Check sheet for the modelled part. Datum: model origin and axes. Units: mm. Face numbers are marked on the shaded views. A direction names the side the tool comes from. Coordinates: 2 decimals unless noted, no trailing zeros. Loops run counter-clockwise (first coordinate to the right, second up) from the corner with the lowest first, then second, coordinate; pieces in that order, holes last. Notation, with made-up numbers: (-21.5, -26.75) - (18.5, -26.75) arc R26 cw to (18.5, -2.75) - close; hole circle Ø4 at (78.5, -36.5). An arc over 180 degrees is marked (long way). Use a Markdown table: item, result. Add a question column.
1) Sectioned sample at C-C, the plane y = 41.5. Enter the section's corners in (x, z) (3 decimals), then the cut area to 3 significant figures.
2) Sectioned sample at D-D, the plane z = 34. Enter the section's corners in (x, y) (3 decimals), then the cut area to 3 significant figures.
3) Thickness scan on line 1 (Y direction, x = 21.5, z = 5); line 2 (Z direction, x = 13.75, y = 14) (3 decimals); line 3 (X direction, y = 38.5, z = 10) (3 decimals). Record the ranges inside material, lowest first.
4) Go/stop test with flat-tipped pins: P1, Ø5, axis at y = 5, z = 23.5, coming from the -X side; P2, Ø12, axis at y = 36, z = 15, coming from the +X side (3 decimals); P3, Ø12.5, axis at x = 15.5, y = 23, coming from the +Z side; P4, Ø1.6, axis at y = -2, z = 38, coming from the +X side (3 decimals). Record where each tip stops, or that it passes through.
5) Sectioned sample at B-B, the plane z = 51. Enter the section's corners in (x, y) (3 decimals), then the cut area to 3 significant figures.
6) Tool access check on the marked faces 1 and 2. Record the directions out of +Z, -Z, +X, -X, +Y, -Y that give a thin tool (end or side, any length) a straight path to the whole face; none if there is none.
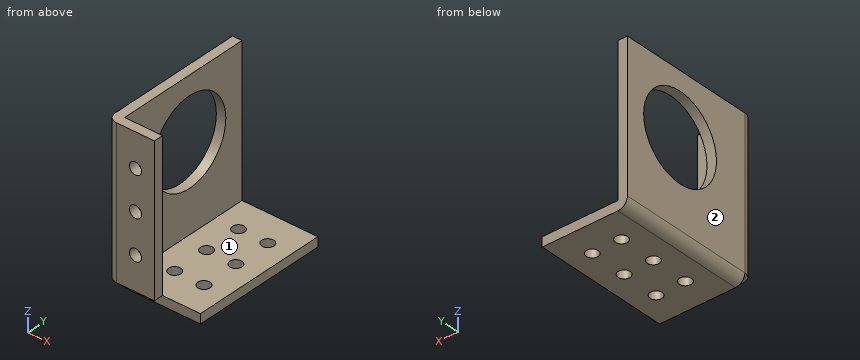
Autodesk Inventor part; units mm, degrees
ref_plane "YZ Plane" through (0, 0, 0) normal (1, 0, 0) x (0, 1, 0)
ref_plane "XZ Plane" through (0, 0, 0) normal (0, 1, 0) x (-1, 0, 0)
ref_plane "XY Plane" through (0, 0, 0) normal (0, 0, 1) x (1, 0, 0)
sketch "Sketch1" plane through (0, 0, 0) normal (1, 0, 0) x (0, 1, 0)
  line L0 (0, 0) -> (46.0357, 0)
  line L1 (46.0357, 0) -> (46.0357, -49.1998)
  line L2 (46.0357, -49.1998) -> (0, -49.1998)
  line L3 (0, -49.1998) -> (0, 0)
  circle A0 centre (25.4109, -28.575) radius 14.2748
  point P0 (39.6857, -28.575)
  point P1 (25.4109, -42.8498)
  dimension "d0" = 25.4109
  dimension "d1" = 28.5496
  dimension "d2" = 6.35
  dimension "d3" = 6.35
  dimension "d4" = 28.575
extrude "Extrusion1" add sketch "Sketch1" along normal blind 3.175
sketch "Sketch2" plane through (0, 0, -49.1998) normal (0, -1, 0) x (1, 0, 0)
  line L0 (3.175, 49.1998) -> (3.175, 0)
  line L1 (3.175, 49.1998) -> (15.875, 49.1998)
  line L2 (15.875, 49.1998) -> (15.875, 0)
  line L3 (15.875, 0) -> (3.175, 0)
  line L4 (3.175, 0) -> (3.175, 49.1998)
  point P0 (0, 49.1998)
  dimension "d7" = 12.7
extrude "Extrusion2" add sketch "Sketch2" along normal blind 3.175
sketch "Sketch3" plane through (0, 0, 0) normal (0, 0, 1) x (1, 0, 0)
  line L0 (3.175, 0) -> (3.175, 46.0357)
  line L1 (3.175, 0) -> (28.575, 0)
  line L2 (28.575, 0) -> (28.575, 49.2107)
  line L3 (28.575, 49.2107) -> (3.175, 49.2107)
  line L4 (3.175, 49.2107) -> (3.175, 0)
  point P0 (0, 0)
  dimension "d10" = 25.4
extrude "Extrusion3" add sketch "Sketch3" along normal blind 3.175
sketch "Sketch4" plane through (3.175, -3.175, 0) normal (0, 0, 1) x (1, 0, 0)
  line L0 (-3.175, 3.175) -> (0, 3.175)
  line L1 (0, 3.175) -> (0, 0)
  arc A0 (-3.175, 3.175) -> (0, 0) centre (0, 3.175) ccw
extrude "Extrusion4" add sketch "Sketch4" against normal up to surface (49.1998 mm away)
sketch "Sketch6" plane through (0, 0, 3.175) normal (0, 0, 1) x (1, 0, 0)
  line L0 (3.175, 0) -> (28.575, 0)
  line L1 (28.575, 0) -> (28.575, 49.2107)
  line L2 (28.575, 49.2107) -> (3.175, 49.2107)
  circle A0 centre (10.9643, 35.5428) radius 2.032
  circle A1 centre (20.7857, 35.5428) radius 2.032
  line L3 (12.9963, 35.5428) -> (18.7537, 35.5428)
  line L4 (8.9323, 35.5428) -> (3.175, 35.5428)
  line L5 (22.8177, 35.5428) -> (28.575, 35.5428)
  circle A2 centre (10.9643, 23.0179) radius 2.032
  circle A3 centre (10.9643, 10.4929) radius 2.032
  line L6 (28.575, 49.2107) -> (3.175, 49.2107)
  line L7 (10.9643, 25.0499) -> (10.9643, 33.5108)
  line L8 (10.9643, 12.5249) -> (10.9643, 20.9859)
  line L9 (10.9643, 8.4609) -> (10.9643, 0)
  circle A4 centre (20.7857, 23.0179) radius 2.032
  circle A5 centre (20.7857, 10.4929) radius 2.032
  line L10 (3.175, 49.2107) -> (3.175, 0)
  line L11 (3.175, 46.0357) -> (28.575, 46.0357)
  line L12 (10.9643, 37.5748) -> (10.9643, 46.0357)
  point P0 (0, 0)
  dimension "d17" = 4.064
  dimension "d20" = 4.064
  dimension "d23" = 4.064
  dimension "d24" = 4.064
  dimension "d25" = 4.064
  dimension "d26" = 4.064
  dimension "d34" = 3.175
extrude "Extrusion6" cut sketch "Sketch6" against normal blind 3.175 contours A3 | A0 | A1 | A2 | A4 | A5
sketch "Sketch7" plane through (0, 0, -49.1998) normal (0, 1, 0) x (1, 0, 0)
  line L0 (3.175, -49.1998) -> (15.875, -49.1998)
  line L1 (15.875, -49.1998) -> (15.875, 0) construction
  line L2 (15.875, 0) -> (3.175, 0)
  line L3 (3.175, -49.1998) -> (3.175, 0)
  circle A0 centre (9.525, -11.284) radius 2.032
  circle A1 centre (9.525, -24.5999) radius 2.032
  circle A2 centre (9.525, -37.9158) radius 2.032
  line L4 (9.525, -9.2519) -> (9.525, 0)
  line L5 (9.525, -13.3159) -> (9.525, -22.5679) construction
  line L6 (9.525, -26.6319) -> (9.525, -35.8838)
  line L7 (9.525, -39.9478) -> (9.525, -49.1998)
  line L8 (28.575, -49.1998) -> (3.175, -49.1998)
  point P0 (0, -49.1998)
  dimension "d29" = 4.064
  dimension "d30" = 4.064
  dimension "d31" = 4.064
extrude "Extrusion7" cut sketch "Sketch7" against normal blind 3.175
sketch "Sketch8" plane through (0, 0, 3.175) normal (0, 0, 1) x (1, 0, 0)
  line L0 (3.175, 49.2107) -> (3.175, 46.0357)
  line L1 (28.575, 49.2107) -> (3.175, 49.2107)
  line L2 (3.175, 46.0357) -> (28.575, 46.0357)
  line L3 (28.575, 46.0357) -> (28.575, 49.2107)
  line L4 (28.575, 49.2107) -> (3.175, 49.2107)
  line L5 (3.175, 49.2107) -> (3.175, 46.0357)
  point P0 (0, 0)
extrude "Extrusion8" cut sketch "Sketch8" against normal blind 25.4
sketch "Sketch9" plane through (0, 46.0357, 0) normal (0, 1, 0) x (1, 0, 0)
  line L0 (0, 0) -> (3.175, 0)
  line L1 (3.175, -3.175) -> (3.175, 0)
  arc A0 (0, 0) -> (3.175, -3.175) centre (3.175, 0) ccw
extrude "Extrusion9" add sketch "Sketch9" against normal up to surface (46.0357 mm away)
mirror "Mirror1" about plane through (15.875, 24.6054, 3.175) normal (0, 0, 1)
sketch "Sketch10" plane through (0, 46.0357, -49.1998) normal (0, 1, 0) x (1, 0, 0)
  line L0 (-4.9915, -52.3748) -> (39.2874, -52.3748)
  line L1 (39.2874, -52.3748) -> (39.2874, 13.8222)
  line L2 (39.2874, 13.8222) -> (-4.9915, 13.8222)
  line L3 (-4.9915, 13.8222) -> (-4.9915, -52.3748)
  point P0 (0, -49.1998)
extrude "Extrusion10" cut sketch "Sketch10" against normal blind 53.975
properties part number "Robot to Bottomish Plate to Pivot Hex Axle OTHER SIDE"
Solved:
| question | item | result |
|---|---|---|
| 1 | outline | (0, 6.35) arc R3.175 ccw to (3.175, 3.175) - (28.575, 3.175) - (28.575, 6.35) - (3.175, 6.35) - (3.175, 55.55) - (0, 55.55) - close |
| 1 | area | 245 mm2 |
| 2 | outline | (0, 0) arc R3.175 ccw to (3.175, -3.175) - (15.875, -3.175) - (15.875, 0) - (3.175, 0) - (3.175, 11.166) - (0, 11.166) - close; (0, 39.656) - (3.175, 39.656) - (3.175, 46.036) - (0, 46.036) - close |
| 2 | area | 104 mm2 |
| 3 | line 1 | y = 0 to 8.59, 12.4 to 21.12, 24.92 to 33.64, 37.45 to 46.04 |
| 3 | line 2 | z = 3.175 to 6.35 |
| 3 | line 3 | x = 0 to 3.175 |
| 4 | P1 | stops at x = 0 |
| 4 | P2 | stops at x = 3.175 |
| 4 | P3 | stops at z = 6.35 |
| 4 | P4 | stops at x = 15.875 |
| 5 | outline | (0, 0) arc R3.175 ccw to (3.175, -3.175) - (15.875, -3.175) - (15.875, 0) - (3.175, 0) - (3.175, 46.036) - (0, 46.036) - close |
| 5 | area | 194 mm2 |
| 6 | face 1 | +Z, +X, +Y |
| 6 | face 2 | +Z, -Z, -X, +Y, -Y |
